```python
from build123d import *

# Parameters (mm, degrees)
BOSS_EXTRUDE1_DEPTH = 10
SKETCH2_W           = 10.53641682
SKETCH2_H           = 17
BOSS_EXTRUDE2_DEPTH = 12.5
RIB1_REACH          = 117.825
SKETCH3_WALL_W      = 270.198153966
SKETCH3_WALL_H      = 5
CUT_EXTRUDE1_REACH  = 169.608
SKETCH4_R           = 2.55
CUT_EXTRUDE2_DEPTH  = 3
SKETCH6_R           = 11.1
CUT_EXTRUDE3_DEPTH  = 7
CUT_EXTRUDE5_REACH  = 107.084
SKETCH8_R           = 4.5
SKETCH9_R           = 11.1
CUT_EXTRUDE6_DEPTH  = 7
CUT_EXTRUDE7_REACH  = 107.084
SKETCH10_R          = 4.5
SKETCH12_R          = 2.05
CUT_EXTRUDE9_DEPTH  = 105.684048451
CUT_EXTRUDE10_DEPTH = 3
CUT_EXTRUDE11_REACH = 108.343
CUT_EXTRUDE12_REACH = 108.343
SKETCH16_W          = 53
SKETCH16_H          = 93.98301549
CUT_EXTRUDE13_DEPTH = 5
FILLET3_R           = 4
SKETCH17_W          = 12
SKETCH17_H          = 3
BOSS_EXTRUDE3_DEPTH = 5
SKETCH18_W          = 12
SKETCH18_H          = 2
BOSS_EXTRUDE4_DEPTH = 8
RIB2_REACH          = 144.796
SKETCH19_WALL_W     = 294.663434656
SKETCH19_WALL_H     = 12


with BuildPart() as part:
    # Sketch1 → Boss-Extrude1 (new body)
    with BuildSketch(Plane(origin=(0, 0, 0), x_dir=(1, 0, 0), z_dir=(0, 1, 0))):
        with BuildLine():
            Line((-74, 26.5), (74, 26.5))
            ThreePointArc((74, 26.5), (100.5, 0), (74, -26.5))
            Line((74, -26.5), (-74, -26.5))
            Line((-74, -26.5), (-74, 26.5))
        make_face()
    extrude(amount=BOSS_EXTRUDE1_DEPTH)

    # Sketch2 → Boss-Extrude2 (add)
    with BuildSketch(Plane(origin=(0, 10, 0), x_dir=(1, 0, 0), z_dir=(0, 1, 0))):
        with Locations((-68.73179159, -18)):
            Rectangle(SKETCH2_W, SKETCH2_H)
    boss_extrude2 = extrude(amount=BOSS_EXTRUDE2_DEPTH)

    # Sketch3 wall → Rib1 (add, up to next)
    with BuildSketch(Plane(origin=(-46.291849308, 16.25, 26.5), x_dir=(0.939692620789, -0.342020143318, 0), z_dir=(0.342020143318, 0.939692620789, 0)), mode=Mode.PRIVATE) as rib1_sk1:
        with Locations((0, 2.5)):
            Rectangle(SKETCH3_WALL_W, SKETCH3_WALL_H)
    rib1_tool1 = extrude(rib1_sk1.sketch, amount=-RIB1_REACH, mode=Mode.PRIVATE) - part.part
    rib1 = rib1_tool1.solids().sort_by_distance((-46.291849308, 16.25, 26.5))[0]
    add(rib1)

    # Sketch4 → Cut-Extrude1 (cut, up to next)
    with BuildSketch(Plane(origin=(-63.46358318, 0, 0), x_dir=(0, 0, -1), z_dir=(1, 0, 0)), mode=Mode.PRIVATE) as cut_extrude1_sk1:
        with Locations((-14.5, 16.25)):
            Circle(SKETCH4_R)
    cut_extrude1_tool1 = extrude(cut_extrude1_sk1.sketch, amount=-CUT_EXTRUDE1_REACH, mode=Mode.PRIVATE) & part.part
    cut_extrude1 = cut_extrude1_tool1.solids().sort_by_distance((-63.463583, 16.25, 14.5))[0]
    add(cut_extrude1, mode=Mode.SUBTRACT)

    # Sketch5 → Cut-Extrude2 (cut)
    with BuildSketch(Plane(origin=(-63.46358318, 0, 0), x_dir=(0, 0, -1), z_dir=(1, 0, 0))):
        Polygon((-10.45, 13.91173141), (-10.45, 18.58826859), (-14.5, 20.92653718), (-18.55, 18.58826859), (-18.55, 13.91173141), (-14.5, 11.57346282), align=None)
    cut_extrude2 = extrude(amount=-CUT_EXTRUDE2_DEPTH, mode=Mode.SUBTRACT)

    # Mirror1: Boss-Extrude2, Rib1, Cut-Extrude1, Cut-Extrude2 across plane
    add(boss_extrude2.mirror(Plane.XY))
    add(rib1.mirror(Plane.XY))
    add(cut_extrude1.mirror(Plane.XY), mode=Mode.SUBTRACT)
    add(cut_extrude2.mirror(Plane.XY), mode=Mode.SUBTRACT)

    # Sketch6 → Cut-Extrude3 (cut)
    with BuildSketch(Plane.XZ):
        with Locations(Location((-40.5, 0, 0), (0, 0, 270))):
            Circle(SKETCH6_R)
    extrude(amount=-CUT_EXTRUDE3_DEPTH, mode=Mode.SUBTRACT)

    # Sketch8 → Cut-Extrude5 (cut, up to next)
    with BuildSketch(Plane.XZ.offset(-7), mode=Mode.PRIVATE) as cut_extrude5_sk1:
        with Locations(Location((-40.5, 0, 0), (0, 0, 270))):
            Circle(SKETCH8_R)
    cut_extrude5_tool1 = extrude(cut_extrude5_sk1.sketch, amount=-CUT_EXTRUDE5_REACH, mode=Mode.PRIVATE) & part.part
    add(cut_extrude5_tool1.solids().sort_by_distance((-40.5, 7, 0))[0], mode=Mode.SUBTRACT)

    # Sketch9 → Cut-Extrude6 (cut)
    with BuildSketch(Plane.XZ):
        with Locations(Location((17, 0, 0), (0, 0, 270))):
            Circle(SKETCH9_R)
    extrude(amount=-CUT_EXTRUDE6_DEPTH, mode=Mode.SUBTRACT)

    # Sketch10 → Cut-Extrude7 (cut, up to next)
    with BuildSketch(Plane.XZ.offset(-7), mode=Mode.PRIVATE) as cut_extrude7_sk1:
        with Locations(Location((17, 0, 0), (0, 0, 270))):
            Circle(SKETCH10_R)
    cut_extrude7_tool1 = extrude(cut_extrude7_sk1.sketch, amount=-CUT_EXTRUDE7_REACH, mode=Mode.PRIVATE) & part.part
    add(cut_extrude7_tool1.solids().sort_by_distance((17, 7, 0))[0], mode=Mode.SUBTRACT)

    # Sketch12 → Cut-Extrude9 (cut, through all)
    with BuildSketch(Plane(origin=(0, 10, 0), x_dir=(1, 0, 0), z_dir=(0, 1, 0))):
        with Locations(Location((1, 20.5, 0), (0, 0, 270))):
            Circle(SKETCH12_R)
        with Locations(Location((31, 20.5, 0), (0, 0, 270))):
            Circle(SKETCH12_R)
    cut_extrude9 = extrude(amount=-CUT_EXTRUDE9_DEPTH, mode=Mode.SUBTRACT)

    # Sketch13 → Cut-Extrude10 (cut)
    with BuildSketch(Plane.XZ):
        Polygon((4.64766982, -22.61135933), (4.652325726, -18.396704937), (1.004655907, -16.285345607), (-2.64766982, -18.38864067), (-2.652325726, -22.603295063), (0.995344093, -24.714654393), align=None)
        Polygon((34.557933518, -22.759301311), (34.735579089, -18.548389844), (31.177645571, -16.289088533), (27.442066482, -18.240698689), (27.264420911, -22.451610156), (30.822354429, -24.710911467), align=None)
    cut_extrude10 = extrude(amount=-CUT_EXTRUDE10_DEPTH, mode=Mode.SUBTRACT)

    # Mirror2: Cut-Extrude9, Cut-Extrude10 across plane
    add(cut_extrude9.mirror(Plane.XY), mode=Mode.SUBTRACT)
    add(cut_extrude10.mirror(Plane.XY), mode=Mode.SUBTRACT)

    # Sketch14 → Cut-Extrude11 (cut, up to next)
    with BuildSketch(Plane.XZ, mode=Mode.PRIVATE) as cut_extrude11_sk1:
        with BuildLine():
            Line((-13.507595269, 15.569177398), (-13.507595269, -5.661519054))
            ThreePointArc((-13.507595269, -5.661519054), (-15.057595269, -7.211519054), (-16.607595269, -5.661519054))
            Line((-16.607595269, -5.661519054), (-16.607595269, 15.569177398))
            ThreePointArc((-16.607595269, 15.569177398), (-15.057595269, 17.119177398), (-13.507595269, 15.569177398))
        make_face()
    cut_extrude11_tool1 = extrude(cut_extrude11_sk1.sketch, amount=-CUT_EXTRUDE11_REACH, mode=Mode.PRIVATE) & part.part
    add(cut_extrude11_tool1.solids().sort_by_distance((-15.057595, 0, 4.953829))[0], mode=Mode.SUBTRACT)

    # Sketch15 → Cut-Extrude12 (cut, up to next)
    with BuildSketch(Plane.XZ, mode=Mode.PRIVATE) as cut_extrude12_sk1:
        with BuildLine():
            Line((42.621659424, 20.124694382), (42.621659424, 4.616853199))
            ThreePointArc((42.621659424, 4.616853199), (41.071659424, 3.066853199), (39.521659424, 4.616853199))
            Line((39.521659424, 4.616853199), (39.521659424, 20.124694382))
            ThreePointArc((39.521659424, 20.124694382), (41.071659424, 21.674694382), (42.621659424, 20.124694382))
        make_face()
    cut_extrude12_tool1 = extrude(cut_extrude12_sk1.sketch, amount=-CUT_EXTRUDE12_REACH, mode=Mode.PRIVATE) & part.part
    add(cut_extrude12_tool1.solids().sort_by_distance((41.071659, 0, 12.370774))[0], mode=Mode.SUBTRACT)

    # Sketch16 → Cut-Extrude13 (cut)
    with BuildSketch(Plane(origin=(0, 10, 0), x_dir=(1, 0, 0), z_dir=(0, 1, 0))):
        with Locations((74, 0)):
            Rectangle(SKETCH16_W, SKETCH16_H)
    extrude(amount=-CUT_EXTRUDE13_DEPTH, mode=Mode.SUBTRACT)

    # Fillet3
    fillet3_edges = [part.edges().sort_by_distance(p)[0] for p in [
        (47.5, 10, 0),
    ]]
    fillet(fillet3_edges, radius=FILLET3_R)

    # Sketch17 → Boss-Extrude3 (add)
    with BuildSketch(Plane(origin=(0, 5, 0), x_dir=(1, 0, 0), z_dir=(0, 1, 0))):
        with Locations((58.5, 9)):
            Rectangle(SKETCH17_W, SKETCH17_H)
    extrude(amount=BOSS_EXTRUDE3_DEPTH)

    # Sketch18 → Boss-Extrude4 (add)
    with BuildSketch(Plane(origin=(0, 0, -10.5), x_dir=(-1, 0, 0), z_dir=(0, 0, -1))):
        with Locations((-58.5, 9)):
            Rectangle(SKETCH18_W, SKETCH18_H)
    extrude(amount=BOSS_EXTRUDE4_DEPTH)

    # Sketch19 wall → Rib2 (add, up to next)
    with BuildSketch(Plane(origin=(64.5, 7.5, -5), x_dir=(0, -0.707106781187, 0.707106781187), z_dir=(0, -0.707106781187, -0.707106781187)), mode=Mode.PRIVATE) as rib2_sk1:
        with Locations((0, 6)):
            Rectangle(SKETCH19_WALL_W, SKETCH19_WALL_H)
    rib2_tool1 = extrude(rib2_sk1.sketch, amount=RIB2_REACH, mode=Mode.PRIVATE) - part.part
    add(rib2_tool1.solids().sort_by_distance((64.5, 7.5, -5))[0])


solid = part.part
```
Design review of the part built by this model. Coordinates are the model's own, in mm. A direction names the side the tool comes from. Give positions to 0.01 mm unless a question says otherwise; leave off trailing zeros. Write each loop counter-clockwise with the first axis right and the second up, starting at its lowest first coordinate (ties: lowest second). Pieces come first, ordered by that corner, then holes. Notation, with made-up numbers: (31, 30) -> (44, 30) arc R18 ccw to (44, 42) -> close; hole circle Ø7 at (8, -21). An arc over 180 degrees is marked (long way). Answer in a Markdown table with one row per item.
(1) Consider section C-C (x = 67.5). State the section outline as (y, z) points, then the cut area to 3 significant figures.
Results:
| item | result |
|---|---|
| outline | (0, -26.5) -> (5, -26.5) -> (5, 26.5) -> (0, 26.5) -> close |
| area | 265 mm2 |
(2) Consider section B-B (x = 11). State the section outline as (y, z) points.
Results:
| item | result |
|---|---|
| outline | (0, -26.5) -> (10, -26.5) -> (10, 26.5) -> (0, 26.5) -> (0, 9.34) -> (7, 9.34) -> (7, -9.34) -> (0, -9.34) -> close |
(3) Clearance check with flat-ended pins moving along their axes: pin 1 (2.5 mm diameter, centred on x = 59, y = 6.5, fed in from -Z); pin 2 (10 mm diameter, centred on x = -33, z = -12.5, fed in from +Y); pin 3 (8 mm diameter, centred on x = 75, z = 3, fed in from +Y). State where each tip first meets the part, or that it passes through.
Results:
| item | result |
|---|---|
| pin 1 | z = -10.5 |
| pin 2 | y = 10 |
| pin 3 | y = 5 |
(4) Mouldability with a two-part tool opening along X and no side actions: class faces 5 (the flat face through (-65, 16, -18.55)), 6 (the flat face through (-16.608, 5, 5)), 7 (the flat face through (-66.464, 14, 13)) as +X half, -X half, draft (parallel to the pull), parting line (faces both ways), or undercut.
Results:
| item | result |
|---|---|
| face 5 | draft |
| face 6 | undercut |
| face 7 | +X half |
(5) Consider section A-A (z = 0). State the section outline as (x, y) points.
Results:
| item | result |
|---|---|
| outline | (-74, 0) -> (-51.6, 0) -> (-51.6, 7) -> (-45, 7) -> (-45, 10) -> (-74, 10) -> close; (-36, 7) -> (-29.4, 7) -> (-29.4, 0) -> (-16.61, 0) -> (-16.61, 10) -> (-36, 10) -> close; (-13.51, 0) -> (5.9, 0) -> (5.9, 7) -> (12.5, 7) -> (12.5, 10) -> (-13.51, 10) -> close; (21.5, 7) -> (28.1, 7) -> (28.1, 0) -> (100.5, 0) -> (100.5, 5) -> (47.5, 5) -> (47.5, 6) arc R4 ccw to (43.5, 10) -> (21.5, 10) -> close |
(6) For faces 1 (the flat face through (39.522, 5, 12)), 2 (the flat face through (52.5, 7, -10)), 3 (the flat face through (58, 6, -10.5)), 4 (the flat face through (-65, 16, 18.55)), list the 3-axis set-ups (+Z, -Z, +X, -X, +Y, -Y) from which the entire face can be reached by the end or side of a thin tool; tool diameter is ignored.
Results:
| item | result |
|---|---|
| face 1 | +Y, -Y |
| face 2 | +Z, -Z, +Y |
| face 3 | -Z, +X |
| face 4 | +X |
(7) To check wall thickness, follow probe 1 along X at (y, z) = (3, 0); probe 2 along X at (y, z) = (7.65, 0); probe 3 along X at (y, z) = (8, -20.5). State the ranges of each line that lie inside material, in increasing order.
Results:
| item | result |
|---|---|
| probe 1 | -74 to -51.6, -29.4 to -16.61, -13.51 to 5.9, 28.1 to 100.5 |
| probe 2 | -74 to -45, -36 to -16.61, -13.51 to 12.5, 21.5 to 47.14 |
| probe 3 | -74 to -1.05, 3.05 to 28.95, 33.05 to 46.96 |
